Verification items for the finished model (mm, model axes). Give positions to 0.01 mm unless a question says otherwise; leave off trailing zeros. Order: outer loops, then holes, each group sorted by start corner. A loop starts at its lowest first (then second) coordinate and runs counter-clockwise, first axis right, second up. Notation, with made-up numbers: (49.25, 48) - (92.25, 48) arc R11 cw to (92.25, 57) - close; hole circle Ø7 at (9.5, 65.5). An arc over 180 degrees is marked (long way). Answer as a JSON object with one key per item and string values. Group by question number.
(1) Depth check by flat-ended pin: pin 1 Ø2 at (x, z) = (-118.46, 0) entering from -Y. Enter the tip coordinate at first touch or a pass-through.
(2) Thickness scan on line 1 (Z direction, x = -73.5, y = 1.25); line 2 (X direction, y = 2.25, z = -16.5); line 3 (Z direction, x = -13, y = 2.15) (3 decimals). Record the ranges inside material, lowest first.
(3) Section check B-B (y = 1.1). Count the separate pieces of the cut face and the enclosed holes in it, then the cut area to 3 significant figures.
(4) Section check C-C (z = 14). Record the boundary of the cut face in (x, y), then the cut area to 3 significant figures.
(5) Section check A-A (x = -13). Record the boundary of the cut face in (y, z) (3 decimals).
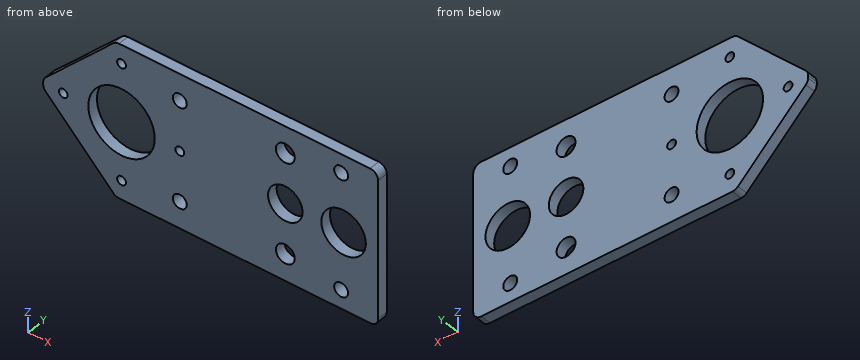
```python
from build123d import *

# Parameters (mm, degrees)
SKETCH1_R           = 8.375
SKETCH1_R_2         = 3.56
SKETCH1_R_3         = 2.625
SKETCH1_R_4         = 12.5
SKETCH1_R_5         = 1.65
SKETCH1_R_6         = 6.5
BOSS_EXTRUDE1_DEPTH = 4.064


with BuildPart() as part:
    # Sketch1 → Boss-Extrude1 (new body)
    with BuildSketch(Plane.XZ):
        with BuildLine():
            Line((0, -26), (0, 26))
            ThreePointArc((0, 26), (-0.878679656, 28.121320344), (-3, 29))
            Line((-3, 29), (-97.5, 29))
            ThreePointArc((-97.5, 29), (-98.648050297, 28.771638598), (-99.621320344, 28.121320344))
            Line((-99.621320344, 28.121320344), (-125.121320344, 2.621320344))
            ThreePointArc((-125.121320344, 2.621320344), (-125.771638598, 1.648050297), (-126, 0.5))
            Line((-126, 0.5), (-126, -0.5))
            ThreePointArc((-126, -0.5), (-125.771638598, -1.648050297), (-125.121320344, -2.621320344))
            Line((-125.121320344, -2.621320344), (-99.621320344, -28.121320344))
            ThreePointArc((-99.621320344, -28.121320344), (-98.648050297, -28.771638598), (-97.5, -29))
            Line((-97.5, -29), (-3, -29))
            ThreePointArc((-3, -29), (-0.878679656, -28.121320344), (0, -26))
        make_face()
        with Locations((-13, 0)):
            Circle(SKETCH1_R, mode=Mode.SUBTRACT)
        with Locations((-34.92008574, 18.9)):
            Circle(SKETCH1_R_2, mode=Mode.SUBTRACT)
        with Locations((-74.62008574, 18.9)):
            Circle(SKETCH1_R_3, mode=Mode.SUBTRACT)
        with Locations((-34.92008574, -18.9)):
            Circle(SKETCH1_R_2, mode=Mode.SUBTRACT)
        with Locations((-74.62008574, -18.9)):
            Circle(SKETCH1_R_3, mode=Mode.SUBTRACT)
        with Locations((-96.540395956, 0)):
            Circle(SKETCH1_R_4, mode=Mode.SUBTRACT)
        with Locations((-74.62008574, 0)):
            Circle(SKETCH1_R_5, mode=Mode.SUBTRACT)
        with Locations((-118.460706173, 0)):
            Circle(SKETCH1_R_5, mode=Mode.SUBTRACT)
        with Locations((-96.540395956, -21.920310217)):
            Circle(SKETCH1_R_5, mode=Mode.SUBTRACT)
        with Locations((-96.540395956, 21.920310217)):
            Circle(SKETCH1_R_5, mode=Mode.SUBTRACT)
        with Locations((-13.92008574, 21.920310217)):
            Circle(SKETCH1_R_3, mode=Mode.SUBTRACT)
        with Locations((-13.92008574, -21.920310217)):
            Circle(SKETCH1_R_3, mode=Mode.SUBTRACT)
        with Locations((-34.92008574, 0)):
            Circle(SKETCH1_R_6, mode=Mode.SUBTRACT)
    extrude(amount=-BOSS_EXTRUDE1_DEPTH)


solid = part.part
```
Solutions:
{
 "1": {"pin 1": "passes through"},
 "2": {"line 1": "z = -29 to -21.27, -16.53 to -1.21, 1.21 to 16.53, 21.27 to 29", "line 2": "x = -111.24 to -75.68, -73.56 to -37.55, -32.29 to 0", "line 3": "z = -29 to -24.379, -19.462 to -8.375, 8.375 to 19.462, 24.379 to 29"},
 "3": {"separate pieces": "1", "enclosed holes": "13", "area": "5,520 mm2"},
 "4": {"outline": "(-113.74, 0) - (0, 0) - (0, 4.06) - (-113.74, 4.06) - close", "area": "462 mm2"},
 "5": {"outline": "(0, -29) - (4.064, -29) - (4.064, -24.379) - (0, -24.379) - close; (0, -19.462) - (4.064, -19.462) - (4.064, -8.375) - (0, -8.375) - close; (0, 8.375) - (4.064, 8.375) - (4.064, 19.462) - (0, 19.462) - close; (0, 24.379) - (4.064, 24.379) - (4.064, 29) - (0, 29) - close"}
}
